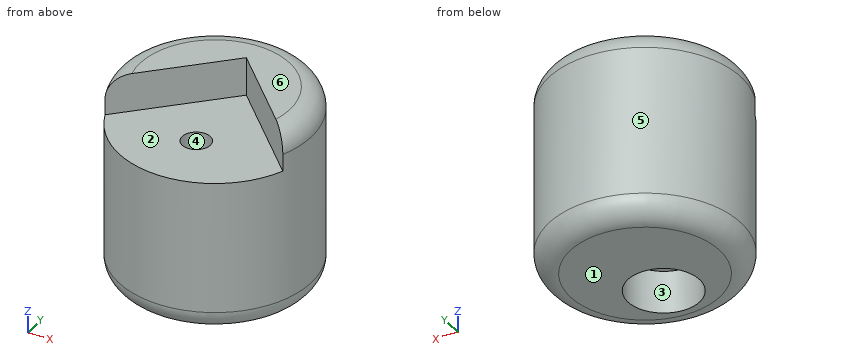
```python
from build123d import *

# Parameters (mm, degrees)
F0_R     = 22.5
F1_DEPTH = 22.5
F3_DEPTH = 9
F4_R     = 5
F5_R     = 5
F7_D     = 6.6
F8_R     = 8.4070446973
F8_R_2   = 3.3
F9_DEPTH = 10


with BuildPart() as f1:
    # F0 (on Top) → F1 (new body, symmetric)
    with BuildSketch(Plane.XY):
        Circle(F0_R)
    extrude(amount=F1_DEPTH, both=True)

    # F2 (on face) → F3 (cut)
    with BuildSketch(Plane.XY.offset(22.5)):
        with BuildLine():
            Line((20.8808748884, -8.3808748884), (0, 12.5))
            Line((0, 12.5), (-20.8808748884, -8.3808748884))
            ThreePointArc((-20.8808748884, -8.3808748884), (0, -22.5), (20.8808748884, -8.3808748884))
        make_face()
    extrude(amount=-F3_DEPTH, mode=Mode.SUBTRACT)

    # F4
    f4_edges = [f1.edges().sort_by_distance(p)[0] for p in [
        (-22.5, 0, -22.5),
    ]]
    fillet(f4_edges, radius=F4_R)

    # F5
    f5_edges = [f1.edges().sort_by_distance(p)[0] for p in [
        (-4.267922, 22.091511, 22.5),
    ]]
    fillet(f5_edges, radius=F5_R)

    # F7 (through all)
    with Locations(Plane.XY.offset(13.5)):
        with Locations((0, -7.456140127)):
            Hole(F7_D / 2)

    # F8 (on face) → F9 (cut)
    with BuildSketch(Plane(origin=(0, 0, -22.5), x_dir=(1, 0, 0), z_dir=(0, 0, -1))):
        with Locations((0, 7.456140127)):
            Circle(F8_R)
        with Locations((0, 7.456140127)):
            Circle(F8_R_2, mode=Mode.SUBTRACT)
    extrude(amount=-F9_DEPTH, mode=Mode.SUBTRACT)


solid = f1.part
```
Can you work these out from the model? Positions are in its coordinate system, mm. Face numbers are marked on the shaded views. A direction names the side the tool comes from. Round coordinates to 2 decimals unless told otherwise and drop trailing zeros. Loops run counter-clockwise (first coordinate to the right, second up) from the corner with the lowest first, then second, coordinate; pieces in that order, holes last.
Item 1: Suppose I cut it at A-A, the plane y = 0. Write out the boundary of the cut face in (x, z), then the cut area to 3 significant figures.
Item 2: Suppose I cut it at C-C, the plane z = -13.5. Write out the boundary of the cut face in (x, y), then the cut area to 3 significant figures.
Item 3: Will these pins go through, and if not, where does the flat tip stop? pin 1 Ø10 at (y, z) = (-3, 13.5) entering from +X; pin 2 Ø2 at (x, y) = (-14.5, -12) entering from -Z; pin 3 Ø10.5 at (x, y) = (0, -7.46) entering from -Z; pin 4 Ø10 at (x, y) = (9.5, -15.5) entering from +Z.
Item 4: Suppose I cut it at B-B, the plane z = -6.5. Write out the boundary of the cut face in (x, y).
Item 5: If we mould it in two halves opening along X, with no side actions, what happens to the marked faces 4, 5 and 6? For each: +X half, -X half, draft (parallel to the pull), parting line (faces both ways), or undercut.
Item 6: Please list where these lines run through material, in increasing order: L1, parallel to Y at x = 0, z = 0; L2, parallel to X at y = 0, z = 17; L3, parallel to Z at x = -11, y = -9.5.
Item 7: Which directions (+Z, -Z, +X, -X, +Y, -Y) give clear straight access to the entire face, cutting with the end or side of a thin tool? Please do the marked faces 1, 2 and 3.
Reported:
1. outline: (-22.5, -17.5) arc R5 ccw to (-17.5, -22.5) - (-3.88, -22.5) - (-3.88, -12.5) - (3.88, -12.5) - (3.88, -22.5) - (17.5, -22.5) arc R5 ccw to (22.5, -17.5) - (22.5, 17.5) arc R5 ccw to (17.5, 22.5) - (12.5, 22.5) - (12.5, 13.5) - (-12.5, 13.5) - (-12.5, 22.5) - (-17.5, 22.5) arc R5 ccw to (-22.5, 17.5) - close
1. area: 1,700 mm2
2. outline: circle Ø45 at (0, 0); hole circle Ø16.81 at (0, -7.46)
2. area: 1,370 mm2
3. pin 1: stops at x = 22.5
3. pin 2: stops at z = -22.49
3. pin 3: stops at z = -12.5
3. pin 4: stops at z = 13.5
4. outline: circle Ø45 at (0, 0); hole circle Ø6.6 at (0, -7.46)
5. face 4: undercut
5. face 5: parting line
5. face 6: draft
6. L1: y = -22.5 to -10.76, -4.16 to 22.5
6. L2: x = -22.5 to -12.5, 12.5 to 22.5
6. L3: z = -22.5 to 13.5
7. face 1: -Z, +X, -X, +Y, -Y
7. face 2: +Z, -Y
7. face 3: -Z
